from build123d import *

# Parameters (mm, degrees)
F0_W     = 50
F0_H     = 4.5
F0_R     = 6.5
F1_DEPTH = 60
F4_W     = 50
F4_H     = 50
F5_DEPTH = 4.5
F6_W     = 50
F6_H     = 65
F6_H_2   = 25
F6_H_3   = 0.5
F7_DEPTH = 60


with BuildPart() as f1:
    # F0 (on Right) → F1 (new body)
    with BuildSketch(Plane.YZ):
        Polygon((-55, 95), (-55, 90), (-50, 90), (-35, 90), (-25, 90), (-15, 90), (0, 90), (5, 90), (5, 95), align=None)
        Polygon((-50, 90), (-55, 90), (-55, -5), (-50, -5), (-50, -4.5), (-50, 0), align=None)
        with Locations((-25, -2.25)):
            Rectangle(F0_W, F0_H)
        Polygon((0, 90), (0, 0), (0, -4.5), (0, -5), (5, -5), (5, 90), align=None)
        with BuildLine():
            ThreePointArc((-15, 80), (-17.9289321881, 87.0710678119), (-25, 90))
            ThreePointArc((-25, 90), (-32.0710678119, 87.0710678119), (-35, 80))
            ThreePointArc((-35, 80), (-25, 70), (-15, 80))
        make_face()
        with Locations((-25, 80)):
            Circle(F0_R, mode=Mode.SUBTRACT)
        with BuildLine():
            Line((-25, 90), (-35, 90))
            Line((-35, 90), (-35, 80))
            ThreePointArc((-35, 80), (-32.0710678119, 87.0710678119), (-25, 90))
        make_face()
        with BuildLine():
            Line((-15, 90), (-25, 90))
            ThreePointArc((-25, 90), (-17.9289321881, 87.0710678119), (-15, 80))
            Line((-15, 80), (-15, 90))
        make_face()
    extrude(amount=F1_DEPTH)

    # F4 (on face) → F5 (cut)
    with BuildSketch(Plane(origin=(0, 0, -4.5), x_dir=(1, 0, 0), z_dir=(0, 0, -1))):
        with Locations((30, 25)):
            Rectangle(F4_W, F4_H)
    extrude(amount=-F5_DEPTH, mode=Mode.SUBTRACT)

    # F6 (on offset) → F7 (cut)
    with BuildSketch(Plane.XZ.offset(55)):
        with Locations((30, 57.5)):
            Rectangle(F6_W, F6_H)
        with Locations((30, 12.5)):
            Rectangle(F6_W, F6_H_2)
        with Locations((30, -4.75)):
            Rectangle(F6_W, F6_H_3)
    extrude(amount=-F7_DEPTH, mode=Mode.SUBTRACT)


solid = f1.part
Input: part model. Units: mm. Frame: model coordinates. A direction names the side the tool comes from. Give positions to 0.01 mm unless a question says otherwise; leave off trailing zeros. Order: outer loops, then holes, each group sorted by start corner. A loop starts at its lowest first (then second) coordinate and runs counter-clockwise, first axis right, second up.
Q1. Section B-B on y = -25. Output: boundary loops of the cut face in (x, z), and give its area (3 significant figures).
Checked values:
outline: (0, -4.5) - (5, -4.5) - (5, 0) - (0, 0) - close; (0, 70) - (5, 70) - (5, 73.5) - (0, 73.5) - close; (0, 86.5) - (5, 86.5) - (5, 90) - (55, 90) - (55, 86.5) - (60, 86.5) - (60, 95) - (0, 95) - close; (55, -4.5) - (60, -4.5) - (60, 0) - (55, 0) - close; (55, 70) - (60, 70) - (60, 73.5) - (55, 73.5) - close
area: 415 mm2
Q2. Section A-A on x = 29.5. Output: boundary loops of the cut face in (y, z), and give its area (3 significant figures).
Checked values:
outline: (-55, -4.5) - (-50, -4.5) - (-50, 0) - (-55, 0) - close; (-55, 90) - (5, 90) - (5, 95) - (-55, 95) - close; (0, -4.5) - (5, -4.5) - (5, 0) - (0, 0) - close
area: 345 mm2
Q3. Section D-D on y = -6. Output: boundary loops of the cut face in (x, z).
Checked values:
outline: (0, -4.5) - (5, -4.5) - (5, 0) - (0, 0) - close; (0, 90) - (60, 90) - (60, 95) - (0, 95) - close; (55, -4.5) - (60, -4.5) - (60, 0) - (55, 0) - close
Q4. Contact query for flat-ended pins moving along their axis: pin 1 Ø4 at (x, y) = (28.5, -41) entering from -Z; pin 2 Ø4 at (x, y) = (3, -14) entering from -Z. Output: stop coordinate, or through.
Checked values:
pin 1: stops at z = 90
pin 2: stops at z = -4.5
Q5. Section C-C on z = 11. Output: boundary loops of the cut face in (x, y), and give its area (3 significant figures).
Checked values:
outline: (0, -55) - (5, -55) - (5, -50) - (0, -50) - close; (0, 0) - (5, 0) - (5, 5) - (0, 5) - close; (55, -55) - (60, -55) - (60, -50) - (55, -50) - close; (55, 0) - (60, 0) - (60, 5) - (55, 5) - close
area: 100 mm2
Q6. Draft query along Y for faces 1 (the flat face through (5, -25, 87)), 2 (the flat face through (2, -50, 44)), 3 (the flat face through (57, -55, 49)). Return one class per face: +Y half, -Y half, draft (parallel to the pull), parting line (faces both ways), or undercut.
Checked values:
face 1: draft
face 2: undercut
face 3: -Y half
Q7. Set-up query: faces 4 (the flat face through (5, -53, 46)), 5 (the flat face through (2, -25, -4.5)), 6 (the flat face through (57, -50, 44)). Return all of +Z, -Z, +X, -X, +Y, -Y with unobstructed straight access to the full face (end or side cutting, diameter ignored); none if empty.
Checked values:
face 4: +Y, -Y
face 5: -Z, +X, -X
face 6: +X, -X
Q8. Ray query, probe 1 along Z at (x, y) = (56.3, -25); probe 2 along Y at (x, z) = (1.9, 80); probe 3 along Y at (x, z) = (4, 79). Return the intervals inside material, ascending.
Checked values:
probe 1: z = -4.5 to 0, 70 to 73.5, 86.5 to 95
probe 2: y = -55 to -50, -35 to -31.5, -18.5 to -15, 0 to 5
probe 3: y = -55 to -50, -34.95 to -31.42, -18.58 to -15.05, 0 to 5
